Design review of the part shown in the three views and the two pictorial views. Dimensions are in mm from the part's minimum x, y and z. Give positions to 0.01 mm unless a question says otherwise; leave off trailing zeros. Loops run counter-clockwise (first coordinate to the right, second up) from the corner with the lowest first, then second, coordinate; pieces in that order, holes last. Notation, with made-up numbers: (67.25, 78.25) -> (101.25, 78.25) arc R12 cw to (101.25, 91.25) -> close; hole circle Ø7 at (7.25, 43). An arc over 180 degrees is marked (long way). Use CSV: the item, a comma, the result in double quotes. Start each with the question number.
Item 1: We need section D-D (y = 0.65). Count the separate pieces of the cut face and the enclosed holes in it, plus the area to 3 significant figures.
Item 2: We need section B-B (z = 5.5). State the section outline as (x, y) points (1 decimal).
Item 3: We need section A-A (x = 25). State the section outline as (y, z) points.
Item 4: Clearance check with flat-ended pins moving along their axes: pin 1 (1.8 mm diameter, centred on x = 34.5, z = 25, fed in from +Y); pin 2 (4 mm diameter, centred on x = 38.79, z = 11.21, fed in from +Y); pin 3 (1 mm diameter, centred on x = 7, y = 0.5, fed in from -Z) (1 decimal); pin 4 (1 mm diameter, centred on x = 41, y = 0.5, fed in from +Z) (1 decimal). State where each tip first meets the part, or that it passes through.
Item 5: We need section C-C (x = 5.5). State the section outline as (y, z) points (1 decimal).
Item 6: Wall thickness on line 1 along X through (y, z) = (1.05, 25); line 2 along Z through (x, y) = (39, 2.1) (1 decimal); line 3 along X through (y, z) = (1, 40) (1 decimal): over which ranges is each line inside the solid? List them lowest first. Write a range as from..to.
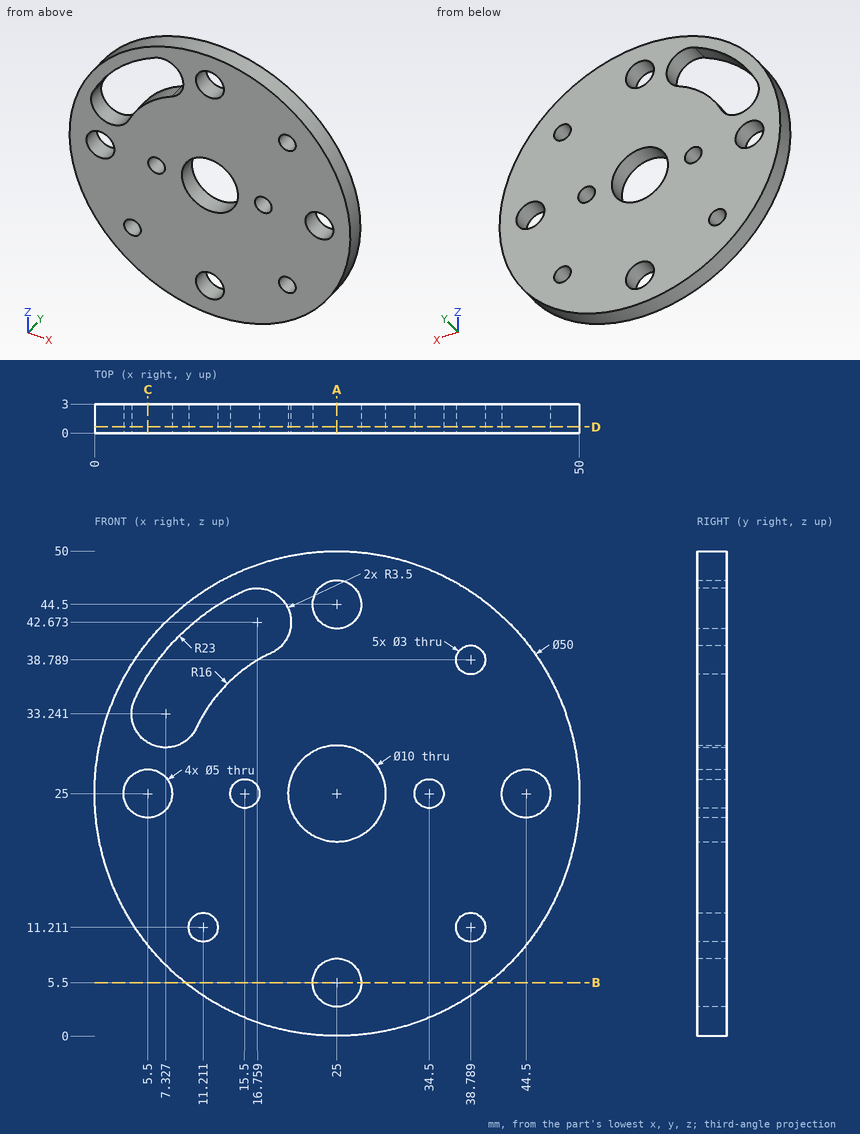
Results found:
1,separate pieces,"1"
1,enclosed holes,"11"
1,area,"1,640 mm²"
2,outline,"(9.4, 0) -> (22.5, 0) -> (22.5, 3) -> (9.4, 3) -> close; (27.5, 0) -> (40.6, 0) -> (40.6, 3) -> (27.5, 3) -> close"
3,outline,"(0, 0) -> (3, 0) -> (3, 3) -> (0, 3) -> close; (0, 8) -> (3, 8) -> (3, 20) -> (0, 20) -> close; (0, 30) -> (3, 30) -> (3, 42) -> (0, 42) -> close; (0, 47) -> (3, 47) -> (3, 50) -> (0, 50) -> close"
4,pin 1,"through"
4,pin 2,"y = 3"
4,pin 3,"z = 7.1"
4,pin 4,"z = 44.6"
5,outline,"(0, 9.4) -> (3, 9.4) -> (3, 22.5) -> (0, 22.5) -> close; (0, 27.5) -> (3, 27.5) -> (3, 30.3) -> (0, 30.3) -> close; (0, 37.2) -> (3, 37.2) -> (3, 40.6) -> (0, 40.6) -> close"
6,line 1,"0..3, 8..14, 17..20, 30..33, 36..42, 47..50"
6,line 2,"4.3..9.7, 12.7..37.3, 40.3..45.7"
6,line 3,"5..7.6, 19..37.9, 39.7..45"
